For this review, take the finished solid that the model builds, in its own axes (mm). A direction names the side the tool comes from. Round coordinates to 2 decimals unless told otherwise and drop trailing zeros. Loops run counter-clockwise (first coordinate to the right, second up) from the corner with the lowest first, then second, coordinate; pieces in that order, holes last.
```python
from build123d import *

# Parameters (mm, degrees)
SKETCH1_R           = 1.375
BOSS_EXTRUDE1_DEPTH = 1.6
SKETCH2_W           = 7.6
SKETCH2_H           = 20
SKETCH2_H_2         = 10
BOSS_EXTRUDE2_DEPTH = 10.15
SKETCH3_W           = 50.6
SKETCH3_H           = 5.1
BOSS_EXTRUDE3_DEPTH = 8.4
SKETCH4_R           = 3.15
BOSS_EXTRUDE4_DEPTH = 7
SKETCH5_W           = 17.5
SKETCH5_H           = 2.5
SKETCH5_W_2         = 10.8
BOSS_EXTRUDE5_DEPTH = 8.4
SKETCH6_W           = 52
SKETCH6_H           = 5
BOSS_EXTRUDE6_DEPTH = 8


with BuildPart() as part:
    # Sketch1 → Boss-Extrude1 (new body)
    with BuildSketch(Plane(origin=(0, 0, 0), x_dir=(1, 0, 0), z_dir=(0, 1, 0))):
        with BuildLine():
            Line((3, 0), (62, 0))
            ThreePointArc((62, 0), (64.121320344, 0.878679656), (65, 3))
            Line((65, 3), (65, 53))
            ThreePointArc((65, 53), (64.121320344, 55.121320344), (62, 56))
            Line((62, 56), (3, 56))
            ThreePointArc((3, 56), (0.878679656, 55.121320344), (0, 53))
            Line((0, 53), (0, 3))
            ThreePointArc((0, 3), (0.878679656, 0.878679656), (3, 0))
        make_face()
        with Locations((3.5, 52.5)):
            Circle(SKETCH1_R, mode=Mode.SUBTRACT)
        with Locations((61.5, 52.5)):
            Circle(SKETCH1_R, mode=Mode.SUBTRACT)
        with Locations((3.5, 3.5)):
            Circle(SKETCH1_R, mode=Mode.SUBTRACT)
        with Locations((61.5, 3.5)):
            Circle(SKETCH1_R, mode=Mode.SUBTRACT)
    extrude(amount=BOSS_EXTRUDE1_DEPTH)

    # Sketch2 → Boss-Extrude2 (add)
    with BuildSketch(Plane(origin=(0, 1.6, 0), x_dir=(1, 0, 0), z_dir=(0, 1, 0))):
        with Locations((6.05, 35)):
            Rectangle(SKETCH2_W, SKETCH2_H)
        with Locations((6.05, 15.7)):
            Rectangle(SKETCH2_W, SKETCH2_H_2)
    extrude(amount=BOSS_EXTRUDE2_DEPTH)

    # Sketch3 → Boss-Extrude3 (add)
    with BuildSketch(Plane(origin=(0, 1.6, 0), x_dir=(1, 0, 0), z_dir=(0, 1, 0))):
        with Locations((32.5, 3.05)):
            Rectangle(SKETCH3_W, SKETCH3_H)
    extrude(amount=BOSS_EXTRUDE3_DEPTH)

    # Sketch4 → Boss-Extrude4 (add)
    with BuildSketch(Plane(origin=(0, 1.6, 0), x_dir=(1, 0, 0), z_dir=(0, 1, 0))):
        with Locations((36.05, 14.35)):
            Circle(SKETCH4_R)
    extrude(amount=BOSS_EXTRUDE4_DEPTH)

    # Sketch5 → Boss-Extrude5 (add)
    with BuildSketch(Plane(origin=(0, 1.6, 0), x_dir=(1, 0, 0), z_dir=(0, 1, 0))):
        with Locations((55.25, 44.85)):
            Rectangle(SKETCH5_W, SKETCH5_H)
        with Locations((58.6, 35.15)):
            Rectangle(SKETCH5_W_2, SKETCH5_H)
        with Locations((58.6, 27.85)):
            Rectangle(SKETCH5_W_2, SKETCH5_H)
    extrude(amount=BOSS_EXTRUDE5_DEPTH)

    # Sketch6 → Boss-Extrude6 (add)
    with BuildSketch(Plane.XZ):
        with Locations((32.5, -52.5)):
            Rectangle(SKETCH6_W, SKETCH6_H)
    extrude(amount=BOSS_EXTRUDE6_DEPTH)


solid = part.part
```
(1) Add section D-D (x = 48). Give the boundary of the cut face in (y, z), plus the area to 3 significant figures.
(2) For L1, parallel to X at y = 1, z = -3.5 (3 decimals); L2, parallel to Z at x = 3.5, y = 0.45 (3 decimals); L3, parallel to Z at x = 9, y = 8.25, list the stretches that pass through material, from the lowest coordinate up.
(3) Add section A-A (y = 4.5). Give the boundary of the cut face in (x, z).
(4) Insertion check: pin 1 Ø10 at (x, z) = (29.5, -19.5) entering from -Y; pin 2 Ø2.5 at (y, z) = (-2, -51.5) entering from -X; pin 3 Ø6.5 at (x, y) = (45, -5.5) entering from +Z. Each pin has a flat end and moves straight along its axis. Give the tip position at first contact, or say it passes through.
(5) The part is to be moulded in two halves that separate along X. For faces 1 (the flat face through (53.2, 6, -35)), 2 (the flat face through (32, 0, -28)), 3 (the cylindrical face through (64.14, 0.79, -55.1)), 4 (the cylindrical face through (4.77, 0.79, -2.97)), say which applies: pulls with the +X half, pulls with the -X half, needs draft (parallel to the pull), parting line crosses it, or undercut.
(6) For faces 5 (the flat face through (32, -4, -50)), 6 (the flat face through (2.25, 7, -16)), 7 (the flat face through (6, 7, -25)), 8 (the flat face through (36, 8.6, -14)), 9 (the flat face through (6, 7, -45)), list the 3-axis set-ups (+Z, -Z, +X, -X, +Y, -Y) from which the entire face can be reached by the end or side of a thin tool; tool diameter is ignored.
(7) Add section C-C (z = -14.35). Give the boundary of the cut face in (x, y), plus the area to 3 significant figures.
(8) Add section B-B (x = 17.5). Give the boundary of the cut face in (y, z).
Outcome:
1. outline: (-8, -55) - (0, -55) - (0, -56) - (1.6, -56) - (1.6, -46.1) - (10, -46.1) - (10, -43.6) - (1.6, -43.6) - (1.6, -5.6) - (10, -5.6) - (10, -0.5) - (1.6, -0.5) - (1.6, 0) - (0, 0) - (0, -50) - (-8, -50) - close
1. area: 193 mm2
2. L1: x = 0 to 2.125, 4.875 to 60.125, 62.875 to 65
2. L2: z = -56 to -53.875, -51.125 to -4.875, -2.125 to 0
2. L3: z = -45 to -25, -20.7 to -10.7, -5.6 to -0.5
3. outline: (2.25, -45) - (9.85, -45) - (9.85, -25) - (2.25, -25) - close; (2.25, -20.7) - (9.85, -20.7) - (9.85, -10.7) - (2.25, -10.7) - close; (7.2, -5.6) - (57.8, -5.6) - (57.8, -0.5) - (7.2, -0.5) - close; circle Ø6.3 at (36.05, -14.35); (46.5, -46.1) - (64, -46.1) - (64, -43.6) - (46.5, -43.6) - close; (53.2, -36.4) - (64, -36.4) - (64, -33.9) - (53.2, -33.9) - close; (53.2, -29.1) - (64, -29.1) - (64, -26.6) - (53.2, -26.6) - close
4. pin 1: stops at y = 0
4. pin 2: stops at x = 6.5
4. pin 3: stops at z = -50
5. face 1: undercut
5. face 2: needs draft
5. face 3: pulls with the +X half
5. face 4: undercut
6. face 5: +Z, +X, -X, -Y
6. face 6: +Z, -Z, -X, +Y
6. face 7: +X, -X, +Y
6. face 8: -Z, +X, +Y
6. face 9: -Z, -X, +Y
7. outline: (0, 0) - (65, 0) - (65, 1.6) - (39.2, 1.6) - (39.2, 8.6) - (32.9, 8.6) - (32.9, 1.6) - (9.85, 1.6) - (9.85, 11.75) - (2.25, 11.75) - (2.25, 1.6) - (0, 1.6) - close
7. area: 225 mm2
8. outline: (-8, -55) - (0, -55) - (0, -56) - (1.6, -56) - (1.6, -5.6) - (10, -5.6) - (10, -0.5) - (1.6, -0.5) - (1.6, 0) - (0, 0) - (0, -50) - (-8, -50) - close
